The listing builds one solid part. Answer for the finished solid, in the listing's coordinates (mm). A direction names the side the tool comes from. Round coordinates to 2 decimals unless told otherwise and drop trailing zeros. Write each loop counter-clockwise with the first axis right and the second up, starting at its lowest first coordinate (ties: lowest second). Pieces come first, ordered by that corner, then holes. Notation, with made-up numbers: M 80,55.5 L 121,55.5 A37 ccw 121,92.5 Z; hole C -2,-37 d9. An arc over 180 degrees is marked long. One line per item, written item: value. Start each with the question number.
(1) Section D-D (z = 1.25) is taken. State how many separate pieces and enclosed holes the cut face has, plus the area to 3 significant figures.
(2) Section B-B (y = -6.75) is taken. Determine the outline of the cut face in (x, z).
(3) Section A-A (x = 41) is taken. Determine the outline of the cut face in (y, z), plus the area to 3 significant figures.
(4) Section C-C (x = 25.5) is taken. Determine the outline of the cut face in (y, z).
(5) For a pull along Y with two mould halves and no side action, classify faces 4 (the cylindrical face through (-20.48, -8.95, 3.45)), 5 (the cylindrical face through (-24.7, -16.2, 3.5)), 6 (the cylindrical face through (43.248, 0.099, 3.451)), 7 (the flat face through (-7, -15.9, 7.2)) as released by +Y, released by -Y, zero draft, split by the parting line, or undercut.
(6) Consider probe 1 along X at (y, z) = (-14.5, 3.5); probe 2 along X at (y, z) = (-0.75, 5.5); probe 3 along Y at (x, z) = (-41, 3). Determine where each line is inside the solid, lowest interval first.
(7) Given P1, Ø0.6, axis at y = -10.5, z = 4, coming from the +X side; P2, Ø3, axis at x = -15.5, z = 6, coming from the +Y side; P3, Ø4, axis at x = 17, z = 7, coming from the +Y side; P4, Ø5.5, axis at x = 1, z = 2.5, coming from the -Y side, each flat-ended and moving along its own axis, determine where each tip first touches the part or whether it passes through.
(8) For faces 1 (the cylindrical face through (35.99, -3.23, 3.45)), 2 (the flat face through (-23, -12, 0)), 3 (the flat face through (-22, -18, 3)), determine the directions among +Z, -Z, +X, -X, +Y, -Y from which every point of the face is accessible in a straight line to the end or side of a thin tool.
```python
from build123d import *

# Parameters (mm, degrees)
SKETCH1_R           = 2.25
BOSS_EXTRUDE2_DEPTH = 7
SKETCH4_W           = 11
SKETCH4_H           = 14
SKETCH4_W_2         = 7
SKETCH4_H_2         = 10
BOSS_EXTRUDE3_DEPTH = 7
SKETCH5_R           = 4
CUT_EXTRUDE1_DEPTH  = 11


with BuildPart() as part:
    # Sketch1 → Boss-Extrude2 (new body)
    with BuildSketch(Plane.XY):
        with BuildLine():
            Line((0, -11.090956097), (0, -13.090956097))
            Line((0, -13.090956097), (0, -15.090956097))
            Line((0, -15.090956097), (0, -17.090956097))
            Line((0, -17.090956097), (0, -19.090956097))
            Line((0, -19.090956097), (0, -21.090956097))
            ThreePointArc((0, -21.090956097), (-11.05703676, -20.528689096), (-22, -18.847688905))
            Line((-22, -18.847688905), (-22, -16.804852023))
            ThreePointArc((-22, -16.804852023), (-24.758641092, -16.187112084), (-27.5, -15.496710289))
            Line((-27.5, -15.496710289), (-27.5, -13.425797094))
            ThreePointArc((-27.5, -13.425797094), (-30.261321018, -12.635734431), (-33, -11.770442452))
            Line((-33, -11.770442452), (-33, -9.661443438))
            ThreePointArc((-33, -9.661443438), (-35.158670825, -8.904528832), (-37.3, -8.099861934))
            Line((-37.3, -8.099861934), (-37.3, -5.951011498))
            ThreePointArc((-37.3, -5.951011498), (-40.012264818, -4.827241682), (-42.690721649, -3.625115213))
            ThreePointArc((-42.690721649, -3.625115213), (-43.149082758, 3.373639474), (-37, 0))
            ThreePointArc((-37, 0), (-35.962178278, -3.272189532), (-33.228136882, -5.348078717))
            ThreePointArc((-33.228136882, -5.348078717), (-16.860380491, -9.644672426), (0, -11.090956097))
        make_face()
        with Locations((-41, 0)):
            Circle(SKETCH1_R, mode=Mode.SUBTRACT)
    extrude(amount=BOSS_EXTRUDE2_DEPTH)

    # Mirror1: part across plane


with BuildPart() as part_1:
    add(part.part)
    add(part.part.mirror(Plane(origin=(0, -11.090956097, 7), x_dir=(0, 0, 1), z_dir=(1, 0, 0))))

    # Sketch4 → Boss-Extrude3 (add, symmetric)
    with BuildSketch(Plane(origin=(0, 0, 0), x_dir=(0, 0, -1), z_dir=(1, 0, 0))):
        with Locations((-3.5, -16)):
            Rectangle(SKETCH4_W, SKETCH4_H)
        with Locations((-3.5, -16)):
            Rectangle(SKETCH4_W_2, SKETCH4_H_2, mode=Mode.SUBTRACT)
    extrude(amount=BOSS_EXTRUDE3_DEPTH, both=True)

    # Sketch5 → Cut-Extrude1 (cut)
    with BuildSketch(Plane.XZ.offset(23)):
        with Locations(Location((0, 3.5, 0), (0, 0, 270))):
            Circle(SKETCH5_R)
    extrude(amount=-CUT_EXTRUDE1_DEPTH, mode=Mode.SUBTRACT)


solid = part_1.part
```
Recorded:
1. separate pieces: 1
1. enclosed holes: 3
1. area: 713 mm2
2. outline: M -37.3,0 L -28.99,0 L -28.99,7 L -37.3,7 Z; M 28.99,0 L 37.3,0 L 37.3,7 L 28.99,7 Z
3. outline: M -4.39,0 L -2.25,0 L -2.25,7 L -4.39,7 Z; M 2.25,0 L 4,0 L 4,7 L 2.25,7 Z
3. area: 27.3 mm2
4. outline: M -16.01,0 L -7.75,0 L -7.75,7 L -16.01,7 Z
5. face 4: released by +Y
5. face 5: released by -Y
5. face 6: undercut
5. face 7: zero draft
6. probe 1: x = -27.5 to -4, 4 to 27.5
6. probe 2: x = -44.93 to -43.12, -38.88 to -36.95, 36.95 to 38.88, 43.12 to 44.93
6. probe 3: y = -4.39 to -2.25, 2.25 to 4
7. P1: stops at x = 33
7. P2: stops at y = -9.62
7. P3: stops at y = -9.25
7. P4: stops at y = -23
8. face 1: +Z, -Z, +Y
8. face 2: -Z, -X, +Y, -Y
8. face 3: +Z, -Z, -X, -Y
